The model under review builds one solid part; all positions refer to its coordinate system, in mm. A direction names the side the tool comes from. Round coordinates to 2 decimals unless told otherwise and drop trailing zeros. Loops run counter-clockwise (first coordinate to the right, second up) from the corner with the lowest first, then second, coordinate; pieces in that order, holes last. Notation, with made-up numbers: (21.25, 43.5) -> (49.25, 43.5) arc R26 ccw to (49.25, 58.5) -> close; hole circle Ø4 at (8, 15.25). An arc over 180 degrees is marked (long way). Return JSON: item names as keys, results as strings. Group by question number.
```python
from build123d import *

# Parameters (mm, degrees)
SKETCH1_W               = 29.972
SKETCH1_H               = 23.114
EXTRUDE1_DEPTH          = 11.938
CUT_EXTRUDE1_DEPTH      = 12.938
SKETCH3_W               = 2.27457
SKETCH3_H               = 7.704666667
CUT_EXTRUDE2_DEPTH      = 15.986
CUT_EXTRUDE2_DEPTH_BACK = 15.986
SKETCH4_W               = 28.3845
SKETCH4_H               = 10.3505
CUT_EXTRUDE3_DEPTH      = 0.254
SKETCH5_W               = 1.255132872
SKETCH5_H               = 4.83743
CUT_EXTRUDE4_DEPTH      = 1.524
EXTRUDE2_DEPTH          = 0.635
CUT_EXTRUDE5_DEPTH      = 10.66343


with BuildPart() as part:
    # Sketch1 → Extrude1 (new body)
    with BuildSketch(Plane.XY):
        Rectangle(SKETCH1_W, SKETCH1_H)
    extrude(amount=EXTRUDE1_DEPTH)

    # Sketch2 → Cut-Extrude1 (cut, through all)
    with BuildSketch(Plane.XY.offset(11.938)):
        with BuildLine():
            Line((-9.990666667, 3.852333333), (-9.790853333, 3.852333333))
            ThreePointArc((-9.790853333, 3.852333333), (-10.010454448, 6.185541418), (-9.5329375, 8.479895833))
            Line((-9.5329375, 8.479895833), (-9.5329375, 11.504083333))
            Line((-9.5329375, 11.504083333), (-12.557125, 11.557))
            Line((-12.557125, 11.557), (12.557125, 11.557))
            Line((12.557125, 11.557), (9.5329375, 11.504083333))
            Line((9.5329375, 11.504083333), (9.5329375, 8.479895833))
            ThreePointArc((9.5329375, 8.479895833), (10.010454448, 6.185541418), (9.790853333, 3.852333333))
            Line((9.790853333, 3.852333333), (9.990666667, 3.852333333))
            ThreePointArc((9.990666667, 3.852333333), (0, -6.138333333), (-9.990666667, 3.852333333))
        make_face()
    extrude(amount=-CUT_EXTRUDE1_DEPTH, mode=Mode.SUBTRACT)

    # Sketch3 → Cut-Extrude2 (cut, two sides)
    with BuildSketch(Plane(origin=(0, 0, 0), x_dir=(0, 0, -1), z_dir=(1, 0, 0))) as cut_extrude2_sk:
        with Locations((-10.800715, 7.704666667)):
            Rectangle(SKETCH3_W, SKETCH3_H)
        with Locations((-1.137285, 7.704666667)):
            Rectangle(SKETCH3_W, SKETCH3_H)
    extrude(amount=CUT_EXTRUDE2_DEPTH, mode=Mode.SUBTRACT)
    extrude(cut_extrude2_sk.sketch, amount=-CUT_EXTRUDE2_DEPTH_BACK, mode=Mode.SUBTRACT)

    # Sketch4 → Cut-Extrude3 (cut)
    with BuildSketch(Plane.XZ.offset(11.557)):
        with Locations((0, 5.969)):
            Rectangle(SKETCH4_W, SKETCH4_H)
    extrude(amount=-CUT_EXTRUDE3_DEPTH, mode=Mode.SUBTRACT)

    # Sketch5 → Cut-Extrude4 (cut)
    with BuildSketch(Plane(origin=(0, 11.557, 0), x_dir=(1, 0, 0), z_dir=(0, 1, 0))):
        with Locations((-14.358433564, -5.969)):
            Rectangle(SKETCH5_W, SKETCH5_H)
        with Locations((14.358433564, -5.969)):
            Rectangle(SKETCH5_W, SKETCH5_H)
    extrude(amount=-CUT_EXTRUDE4_DEPTH, mode=Mode.SUBTRACT)

    # Sketch6 → Cut-Revolve1 (revolve, cut)
    with BuildSketch(Plane(origin=(0, 0, 5.969), x_dir=(-1, 0, 0), z_dir=(0, 0, -1)), mode=Mode.PRIVATE) as cut_revolve1_sk:
        Polygon((2.54, -11.303), (0, -11.303), (0, -6.223), (4.445, -6.223), (4.445, -8.763), (2.54, -8.763), align=None)
    revolve(cut_revolve1_sk.sketch.rotate(Axis((0, 0, 5.969), (0, -1, 0)), 270), axis=Axis((0, 0, 5.969), (0, -1, 0)), mode=Mode.SUBTRACT)  # turned: the seam where the file's is

    # Sketch7 → Extrude2 (add, symmetric)
    with BuildSketch(Plane(origin=(0, 0, 5.969), x_dir=(-1, 0, 0), z_dir=(0, 0, -1))):
        with BuildLine():
            Line((4.047558738, -4.067217721), (7.45308183, -1.000870956))
            Line((7.45308183, -1.000870956), (8.209636208, -1.841109717))
            ThreePointArc((8.209636208, -1.841109717), (6.685060845, -3.572178903), (4.804113117, -4.907456482))
            Line((4.804113117, -4.907456482), (4.047558738, -4.067217721))
        make_face()
        with BuildLine():
            Line((-4.047558738, -4.067217721), (-4.804113117, -4.907456482))
            ThreePointArc((-4.804113117, -4.907456482), (-6.685060845, -3.572178903), (-8.209636208, -1.841109717))
            Line((-8.209636208, -1.841109717), (-7.45308183, -1.000870956))
            Line((-7.45308183, -1.000870956), (-4.047558738, -4.067217721))
        make_face()
    extrude(amount=EXTRUDE2_DEPTH, both=True)

    # Sketch8 → Cut-Extrude5 (cut, through all)
    with BuildSketch(Plane.XY.offset(9.66343)):
        Polygon((-9.5329375, 11.53075), (-11.0569375, 11.53075), (-9.5329375, 9.49875), align=None)
        Polygon((9.5329375, 11.53075), (11.0569375, 11.53075), (9.5329375, 9.49875), align=None)
    extrude(amount=-CUT_EXTRUDE5_DEPTH, mode=Mode.SUBTRACT)


solid = part.part
```
1. We need section D-D, the plane y = -2.25. Write out the cut boundary in (x, z).
2. For P1, Ø1.4, axis at x = 14.5, y = 10.5, coming from the +Z side; P2, Ø1, axis at x = -11.5, z = 1.5, coming from the +Y side; P3, Ø6, axis at x = -11.5, y = 9.5, coming from the -Z side; P4, Ø3, axis at x = -6, y = 1, coming from the -Z side, all flat-tipped, find the tip position at first contact; note any pin that passes through.
3. Wall thickness on line 1 (X direction, y = 8.5, z = 6.25); line 2 (Z direction, x = 13.25, y = 8.75); line 3 (X direction, y = -0.5, z = 1.5): over which ranges is each line inside the solid? List them lowest first.
4. Draft analysis for pull direction Z (two halves, no side actions). For faces 1 (the face through (12, 3.852, 1)), 2 (the face through (6, -3, 5.334)), 3 (the face through (2, -8.763, 8)), state which applies: pulls with the +Z half, pulls with the -Z half, needs draft (parallel to the pull), parting line crosses it, or undercut.
5. We need section B-B, the plane x = 0. Write out the cut boundary in (y, z).
6. We need section C-C, the plane z = 3. Write out the cut boundary in (x, y), then the cut area to 3 significant figures.
7. We need section A-A, the plane y = -7.25. Write out the cut boundary in (x, z) (3 decimals).
8. Tool access review of faces 4 (the face through (-1.72, -10.05, 4.1)), 5 (the face through (14, 11, 3.55)), 6 (the face through (12, 3.852, 11)), 7 (the face through (-12, 3.852, 1)), 8 (the face through (-7.83, -1.42, 5.98)): name each direction out of +Z, -Z, +X, -X, +Y, -Y from which nothing blocks a thin tool from reaching the whole face with its end or side.
Check sheet entries:
{
 "1": {"outline": "(-14.99, 0) -> (-7.91, 0) -> (-7.91, 5.33) -> (-6.07, 5.33) -> (-6.07, 6.6) -> (-7.91, 6.6) -> (-7.91, 11.94) -> (-14.99, 11.94) -> close; (6.07, 5.33) -> (7.91, 5.33) -> (7.91, 0) -> (14.99, 0) -> (14.99, 11.94) -> (7.91, 11.94) -> (7.91, 6.6) -> (6.07, 6.6) -> close"},
 "2": {"P1": "stops at z = 9.66", "P2": "stops at y = 3.85", "P3": "stops at z = 2.27", "P4": "passes through"},
 "3": {"line 1": "x = -14.99 to -9.53, 9.53 to 14.99", "line 2": "z = 2.27 to 9.66", "line 3": "x = -14.99 to -8.99, 8.99 to 14.99"},
 "4": {"face 1": "needs draft", "face 2": "pulls with the -Z half", "face 3": "undercut"},
 "5": {"outline": "(-11.56, 0) -> (-6.14, 0) -> (-6.14, 11.94) -> (-11.56, 11.94) -> (-11.56, 11.14) -> (-11.3, 11.14) -> (-11.3, 8.51) -> (-8.76, 8.51) -> (-8.76, 10.41) -> (-6.22, 10.41) -> (-6.22, 1.52) -> (-8.76, 1.52) -> (-8.76, 3.43) -> (-11.3, 3.43) -> (-11.3, 0.79) -> (-11.56, 0.79) -> close"},
 "6": {"outline": "(-14.99, -11.56) -> (-14.19, -11.56) -> (-14.19, -11.3) -> (14.19, -11.3) -> (14.19, -11.56) -> (14.99, -11.56) -> (14.99, 11.56) -> (12.56, 11.56) -> (11.06, 11.53) -> (9.53, 9.5) -> (9.53, 8.48) arc R7.87 cw to (9.79, 3.85) -> (9.99, 3.85) arc R9.99 cw to (-9.99, 3.85) -> (-9.79, 3.85) arc R7.87 cw to (-9.53, 8.48) -> (-9.53, 9.5) -> (-11.06, 11.53) -> (-12.56, 11.56) -> (-14.99, 11.56) -> close; hole (-3.31, -8.76) -> (3.31, -8.76) -> (3.31, -6.22) -> (-3.31, -6.22) -> close", "area": "358 mm²"},
 "7": {"outline": "(-14.986, 0) -> (14.986, 0) -> (14.986, 11.938) -> (-14.986, 11.938) -> close; hole circle Ø8.89 at (0, 5.969)"},
 "8": {"face 4": "-Y", "face 5": "+X, +Y", "face 6": "+Z, +X, -X, +Y", "face 7": "-Z, +X, -X, +Y", "face 8": "+Z, -Z, +Y"}
}
